Design review of the part built by this model. Coordinates are the model's own, in mm. A direction names the side the tool comes from. Give positions to 0.01 mm unless a question says otherwise; leave off trailing zeros. Order: outer loops, then holes, each group sorted by start corner. A loop starts at its lowest first (then second) coordinate and runs counter-clockwise, first axis right, second up. Notation, with made-up numbers: M -28.75,-28.5 L -12.75,-28.5 A20 ccw -12.75,-23.5 Z; hole C 88,-11 d2. An arc over 180 degrees is marked long. Answer as a JSON object with one key per item and string values.
Solid Edge part; units mm, degrees
sketch "Sketch1" plane through (0, 0, 0) normal (0, -1, 0) x (1, 0, 0)
  circle A0 centre (0, 0) radius 18.5
  circle A1 centre (0, 0) radius 20
extrude "Extrusionsausprägung_1" add sketch "Sketch1" against normal blind 136.5
hole "Bohrung_1" at (-20, 10.1, 0) direction (1, 0, 0) diameter 4.2 end up to next
sketch "Sketch2" plane through (-20, 68.25, 0) normal (-1, 0, 0) x (0, -1, 0)
  circle A0 centre (58.15, 0) radius 4
extrude "Extrusionsausschnitt_1" cut sketch "Sketch2" against normal blind 0.5
properties material "Acryl, hoher Anschlag"
(1) We need section A-A (z = 0). Write out the cut boundary in (x, y).
Checked values:
{"outline": "M -20,0 L -18.5,0 L -18.5,8 L -19.5,8 L -19.5,6.1 L -20,6.1 Z; M -20,14.1 L -19.5,14.1 L -19.5,12.2 L -18.5,12.2 L -18.5,136.5 L -20,136.5 Z; M 18.5,0 L 20,0 L 20,136.5 L 18.5,136.5 Z"}
(2) Draft analysis for pull direction Y (two halves, no side actions). For faces 1 (the flat face through (-18, 136.5, -6)), 2 (the cylindrical face through (-18.95, 10.19, -2.1)), 3 (the flat face through (-18, 0, -6)), state which applies: +Y half, -Y half, draft (parallel to the pull), parting line (faces both ways), or undercut.
Checked values:
{"face 1": "+Y half", "face 2": "undercut", "face 3": "-Y half"}
(3) We need section C-C (z = 10.5). Write out the cut boundary in (x, y).
Checked values:
{"outline": "M -17.02,0 L -15.23,0 L -15.23,136.5 L -17.02,136.5 Z; M 15.23,0 L 17.02,0 L 17.02,136.5 L 15.23,136.5 Z"}
(4) We need section B-B (x = 0). Write out the cut boundary in (y, z), plus the area to 4 significant figures.
Checked values:
{"outline": "M 0,-20 L 136.5,-20 L 136.5,-18.5 L 0,-18.5 Z; M 0,18.5 L 136.5,18.5 L 136.5,20 L 0,20 Z", "area": "409.5 mm^2"}
(5) Tool access review of faces 4 (the cylindrical face through (-4.01, 67.29, -18.06)), 5 (the flat face through (-19.5, 12, -2)): name each direction out of +Z, -Z, +X, -X, +Y, -Y from which nothing blocks a thin tool from reaching the whole face with its end or side.
Checked values:
{"face 4": "+Y, -Y", "face 5": "-X"}
(6) We need section D-D (y = 123). Write out the cut boundary in (x, z), plus the area to 3 significant figures.
Checked values:
{"outline": "C 0,0 d40; hole C 0,0 d37", "area": "181 mm^2"}
(7) Insertion check: pin 1 (1 mm diameter, centred on y = 40, z = -12.5, fed in from -X); pin 2 (6 mm diameter, centred on y = 31, z = 3.5, fed in from -X); pin 3 (6 mm diameter, centred on y = 24, z = -11.5, fed in from +X). Each pin has a flat end and moves straight along its axis. Give the tip position at first contact, or say it passes through.
Checked values:
{"pin 1": "stops at x = -16", "pin 2": "stops at x = -19.99", "pin 3": "stops at x = 18.1"}
(8) To check wall thickness, follow L1, parallel to X at y = 29, z = -1; L2, parallel to X at y = 25, z = -9; L3, parallel to Z at x = 12.5, y = 93. State the ranges of each line that lie inside material, in increasing order. Write a range as from..to.
Checked values:
{"L1": "x = -19.97..-18.47, 18.47..19.97", "L2": "x = -17.86..-16.16, 16.16..17.86", "L3": "z = -15.61..-13.64, 13.64..15.61"}
